Answer from the drawing. Dimensions are ordinates in mm from the lowest x, y and z of the part. A direction names the side the tool comes from. Give positions to 0.01 mm unless a question says otherwise; leave off trailing zeros. Loops run counter-clockwise (first coordinate to the right, second up) from the corner with the lowest first, then second, coordinate; pieces in that order, holes last. Notation, with made-up numbers: (26.5, 28) - (85.5, 28) arc R18 cw to (85.5, 37) - close; hole circle Ø9 at (-16.5, 47). An arc over 180 degrees is marked (long way). One line per item, written item: value.
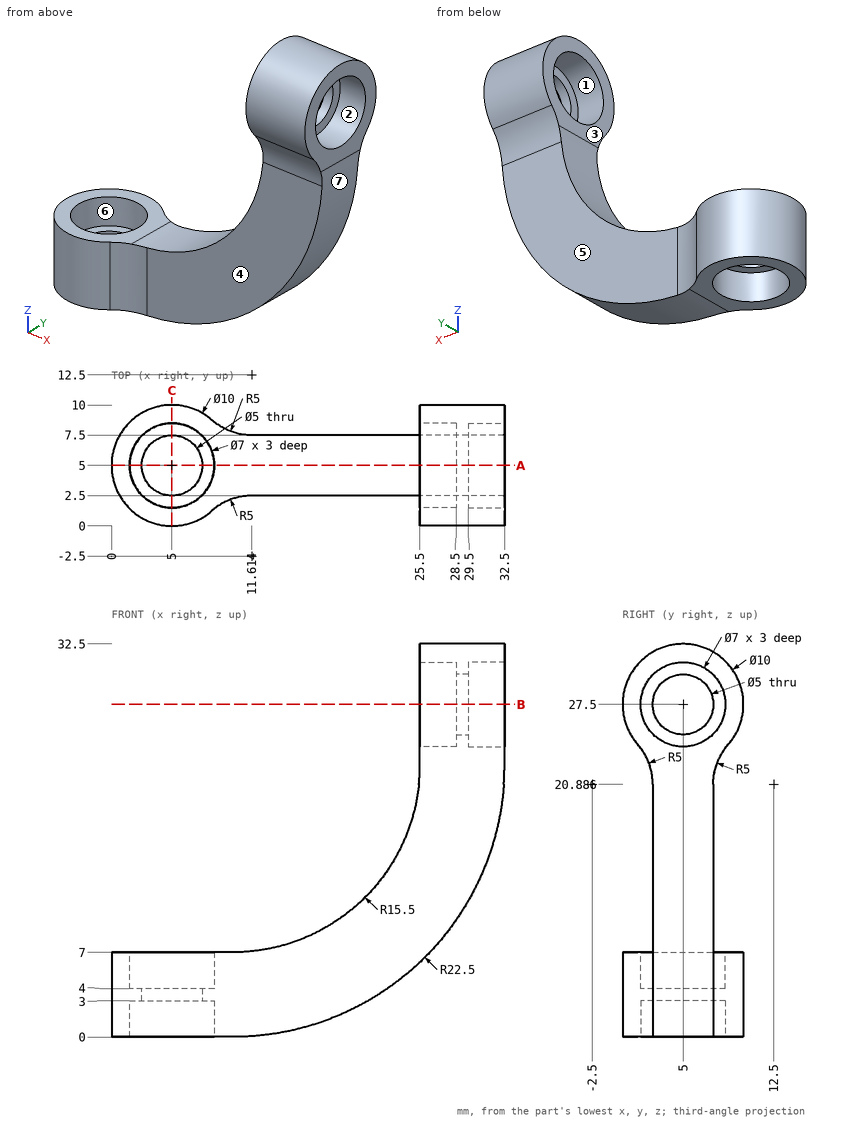
1. Flat-ended cylindrical pins translate along their axes: pin 1 Ø5 at (y, z) = (7, 18) entering from +X; pin 2 Ø5.5 at (y, z) = (5, 27.5) entering from -X; pin 3 Ø6 at (x, y) = (13.5, 7) entering from +Z. Find the tip coordinate at first contact, or state that the pin passes through.
Output:
pin 1: stops at x = 32.41
pin 2: stops at x = 28.5
pin 3: stops at z = 8.43
2. For the marked faces 1, 2, 3 and 4, determine the directions among +Z, -Z, +X, -X, +Y, -Y from which every point of the face is accessible in a straight line to the end or side of a thin tool.
Output:
face 1: -X
face 2: +X
face 3: +Z, -X, +Y, -Y
face 4: -Z, +X, -Y
3. Section B-B (z = 27.5) is taken. Write down the section's boundary in (x, y).
Output:
outline: (25.5, 0) - (32.5, 0) - (32.5, 1.5) - (29.5, 1.5) - (29.5, 2.5) - (28.5, 2.5) - (28.5, 1.5) - (25.5, 1.5) - close; (25.5, 8.5) - (28.5, 8.5) - (28.5, 7.5) - (29.5, 7.5) - (29.5, 8.5) - (32.5, 8.5) - (32.5, 10) - (25.5, 10) - close
4. Section C-C (x = 5) is taken. Write down the section's boundary in (y, z), and give its area (3 significant figures).
Output:
outline: (0, 0) - (1.5, 0) - (1.5, 3) - (2.5, 3) - (2.5, 4) - (1.5, 4) - (1.5, 7) - (0, 7) - close; (7.5, 3) - (8.5, 3) - (8.5, 0) - (10, 0) - (10, 7) - (8.5, 7) - (8.5, 4) - (7.5, 4) - close
area: 23.0 mm²
5. The mould has two halves that part along X. Classify the marked faces 5, 6 and 7: released by +X, released by -X, zero draft, split by the parting line, or undercut.
Output:
face 5: zero draft
face 6: undercut
face 7: released by +X
6. Section A-A (y = 5) is taken. Count the separate pieces of the cut face and the enclosed holes in it, and give its area (3 significant figures).
Output:
separate pieces: 3
enclosed holes: 0
area: 255 mm²
7. Find the intervals of material crossed by line 1 along Y through (x, z) = (5, 3.6); line 2 along X through (y, z) = (6.75, 2) (1 decimal); line 3 along X through (y, z) = (1.25, 26), in increasing order.
Output:
line 1: y = 0 to 2.5, 7.5 to 10
line 2: x = 0.3 to 2, 8 to 19.3
line 3: x = 25.5 to 32.5
